from build123d import *

# Parameters (mm, degrees)
SKETCH1_R           = 5
BOSS_EXTRUDE1_DEPTH = 2.5
SCALE1_SCALE        = 0.3


with BuildPart() as part:
    # Sketch1 → Boss-Extrude1 (new body, symmetric)
    with BuildSketch(Plane.XY):
        with BuildLine():
            Line((-7.5, 0), (-7.5, 50))
            ThreePointArc((-7.5, 50), (0, 57.5), (7.5, 50))
            Line((7.5, 50), (7.5, 0))
            ThreePointArc((7.5, 0), (0, -7.5), (-7.5, 0))
        make_face()
        with Locations((0, 50)):
            Circle(SKETCH1_R, mode=Mode.SUBTRACT)
        with Locations((0, 25)):
            Circle(SKETCH1_R, mode=Mode.SUBTRACT)
        Circle(SKETCH1_R, mode=Mode.SUBTRACT)
    extrude(amount=BOSS_EXTRUDE1_DEPTH, both=True)


with BuildPart() as part_1:
    # Scale1: scaled about (0, 25, 0)
    add(part.part.scale(SCALE1_SCALE).moved(Location((0, 17.5, 0))))


solid = part_1.part
Part model, mm, in its own coordinate system. Give positions to 0.01 mm unless a question says otherwise; leave off trailing zeros. Loops run counter-clockwise (first coordinate to the right, second up) from the corner with the lowest first, then second, coordinate; pieces in that order, holes last. Notation, with made-up numbers: (41.5, 0) -> (70.5, 0) arc R29 cw to (70.5, 29) -> close; hole circle Ø9 at (8, 73.25). An arc over 180 degrees is marked (long way). Write each question's results on one line, items separated by ' | '. Start each with the question number.
Q1. Band-saw the part on A-A on x = 0. List the corners of the cut face in (y, z), plus the area to 4 significant figures.
Q2. Pin check, flat tip, straight feed: P1, Ø2.5, axis at x = 0, y = 25, coming from the +Z side. Stop position of the tip, or through.
Q3. Band-saw the part on D-D on x = -0.85. List the corners of the cut face in (y, z), plus the area to 3 significant figures.
Q4. Band-saw the part on C-C on z = -0.3. List the corners of the cut face in (x, y).
Q5. Wall check: L1, parallel to Y at x = 0, z = 0.4; L2, parallel to Y at x = 0.95, z = 0.1; L3, parallel to X at y = 23.75, z = -0.4. Give the ranges that are in metal, low to high.
Q6. Band-saw the part on B-B on y = 25. List the corners of the cut face in (x, z), plus the area to 3 significant figures.
Q7. Pull direction X, two halves, no side cores. Call faces 1 (the face through (0, 19, 0)), 2 (the face through (2.25, 25, 0)), 3 (the face through (-0.05, 34.75, 0.01)): +X half, -X half, draft (parallel to the pull), parting line (faces both ways), or undercut.
Results are:
1) outline: (15.25, -0.75) -> (16, -0.75) -> (16, 0.75) -> (15.25, 0.75) -> close; (19, -0.75) -> (23.5, -0.75) -> (23.5, 0.75) -> (19, 0.75) -> close; (26.5, -0.75) -> (31, -0.75) -> (31, 0.75) -> (26.5, 0.75) -> close; (34, -0.75) -> (34.75, -0.75) -> (34.75, 0.75) -> (34, 0.75) -> close | area: 15.75 mm²
2) P1: passes through
3) outline: (15.42, -0.75) -> (16.26, -0.75) -> (16.26, 0.75) -> (15.42, 0.75) -> close; (18.74, -0.75) -> (23.76, -0.75) -> (23.76, 0.75) -> (18.74, 0.75) -> close; (26.24, -0.75) -> (31.26, -0.75) -> (31.26, 0.75) -> (26.24, 0.75) -> close; (33.74, -0.75) -> (34.58, -0.75) -> (34.58, 0.75) -> (33.74, 0.75) -> close | area: 17.6 mm²
4) outline: (-2.25, 17.5) arc R2.25 ccw to (2.25, 17.5) -> (2.25, 32.5) arc R2.25 ccw to (-2.25, 32.5) -> close; hole circle Ø3 at (0, 17.5); hole circle Ø3 at (0, 25); hole circle Ø3 at (0, 32.5)
5) L1: y = 15.25 to 16, 19 to 23.5, 26.5 to 31, 34 to 34.75 | L2: y = 15.46 to 16.34, 18.66 to 23.84, 26.16 to 31.34, 33.66 to 34.54 | L3: x = -2.25 to -0.83, 0.83 to 2.25
6) outline: (-2.25, -0.75) -> (-1.5, -0.75) -> (-1.5, 0.75) -> (-2.25, 0.75) -> close; (1.5, -0.75) -> (2.25, -0.75) -> (2.25, 0.75) -> (1.5, 0.75) -> close | area: 2.25 mm²
7) face 1: undercut | face 2: +X half | face 3: parting line
